Solid Edge part; units mm, degrees
sketch "Sketch1" plane through (0, 0, 0) normal (0, -1, 0) x (1, 0, 0)
  line L0 (-7.95, 14.399) -> (-7.95, -6.299)
  arc A0 (-7.95, -6.299) -> (-6.299, -7.95) centre (-6.299, -6.299) ccw
  line L1 (-6.299, -7.95) -> (14.399, -7.95)
  arc A1 (14.399, -7.95) -> (16.05, -6.299) centre (14.399, -6.299) ccw
  line L2 (16.05, -6.299) -> (16.05, 14.399)
  arc A2 (16.05, 14.399) -> (14.399, 16.05) centre (14.399, 14.399) ccw
  line L3 (14.399, 16.05) -> (-6.299, 16.05)
  arc A3 (-6.299, 16.05) -> (-7.95, 14.399) centre (-6.299, 14.399) ccw
  arc A4 (-10.95, -7.648) -> (-7.648, -10.95) centre (-7.648, -7.648) ccw
  line L4 (-7.648, -10.95) -> (15.748, -10.95)
  arc A5 (15.748, -10.95) -> (19.05, -7.648) centre (15.748, -7.648) ccw
  line L5 (19.05, -7.648) -> (19.05, 15.748)
  arc A6 (19.05, 15.748) -> (15.748, 19.05) centre (15.748, 15.748) ccw
  line L6 (15.748, 19.05) -> (-7.648, 19.05)
  arc A7 (-7.648, 19.05) -> (-10.95, 15.748) centre (-7.648, 15.748) ccw
  line L7 (-10.95, 15.748) -> (-10.95, -7.648)
extrude "Protrusion1" add sketch "Sketch1" against normal blind 44.45
properties material "Steel"
Source: CAD feature listing. Evaluate the final solid. Frame: model axes, mm. A direction names the side the tool comes from. Give positions to 0.01 mm unless a question says otherwise; leave off trailing zeros. Write each loop counter-clockwise with the first axis right and the second up, starting at its lowest first coordinate (ties: lowest second). Pieces come first, ordered by that corner, then holes.
1. Section query C-C (y = 18.5). Return the cut outline in (x, z), then the cut area to 3 significant figures.
2. Access query for faces 5 (the face through (4, 0, 18)), 6 (the face through (4, 22, 16.05)). Directions: +Z, -Z, +X, -X, +Y, -Y. A direction counts if a zero-diameter tool reaches every point of the face in a straight line with its end or side. Return the directions, or none.
3. Section query A-A (z = 7). Return the cut outline in (x, y), then the cut area to 3 significant figures.
4. Section query B-B (x = 13). Return the cut outline in (y, z), then the cut area to 3 significant figures.
5. Section query D-D (x = 17). Return the cut outline in (y, z), then the cut area to 3 significant figures.
6. Pull-direction query (X, two-part tool) for faces 1 (the face through (-7.95, 22, 4)), 2 (the face through (18.057, 21.914, -10.008)), 3 (the face through (-10.95, 22, 4)), 4 (the face through (-7.48, 21.91, -7.45)); classes: +X half, -X half, draft (parallel to the pull), parting line (faces both ways), or undercut.
7. Material intervals for line 1 along X through (y, z) = (38.5, 9.5); line 2 along Z through (x, y) = (-7.75, 28.5), sorted ascending.
Output values:
1. outline: (-10.95, -7.65) arc R3.3 ccw to (-7.65, -10.95) - (15.75, -10.95) arc R3.3 ccw to (19.05, -7.65) - (19.05, 15.75) arc R3.3 ccw to (15.75, 19.05) - (-7.65, 19.05) arc R3.3 ccw to (-10.95, 15.75) - close; hole (-7.95, -6.3) arc R1.65 ccw to (-6.3, -7.95) - (14.4, -7.95) arc R1.65 ccw to (16.05, -6.3) - (16.05, 14.4) arc R1.65 ccw to (14.4, 16.05) - (-6.3, 16.05) arc R1.65 ccw to (-7.95, 14.4) - close
1. area: 317 mm2
2. face 5: +Z, -Z, +X, -X, -Y
2. face 6: +Y, -Y
3. outline: (-10.95, 0) - (-7.95, 0) - (-7.95, 44.45) - (-10.95, 44.45) - close; (16.05, 0) - (19.05, 0) - (19.05, 44.45) - (16.05, 44.45) - close
3. area: 267 mm2
4. outline: (0, -10.95) - (44.45, -10.95) - (44.45, -7.95) - (0, -7.95) - close; (0, 16.05) - (44.45, 16.05) - (44.45, 19.05) - (0, 19.05) - close
4. area: 267 mm2
5. outline: (0, -10.7) - (44.45, -10.7) - (44.45, 18.8) - (0, 18.8) - close
5. area: 1,310 mm2
6. face 1: undercut
6. face 2: +X half
6. face 3: -X half
6. face 4: undercut
7. line 1: x = -10.95 to -7.95, 16.05 to 19.05
7. line 2: z = -10.95 to -7.09, 15.19 to 19.05
